Geometry: see drawing. Coordinates: mm, zero at the bounding-box minimum. Round coordinates to 2 decimals unless told otherwise and drop trailing zeros. Loops run counter-clockwise (first coordinate to the right, second up) from the corner with the lowest first, then second, coordinate; pieces in that order, holes last. Notation, with made-up numbers: (73, 59) - (107, 59) arc R24 ccw to (107, 70) - close; hole circle Ø9 at (18, -28.75). An arc over 180 degrees is marked (long way). Use CSV: the item, a comma, the result in double quotes. Start each with the question number.
1. Cut plane B-B (x = 3.25). Return loops of the section in (y, z) (1 decimal).
2. Pull-direction query (Y, two-part tool) for the marked faces 1, 2 and 3; classes: +Y half, -Y half, draft (parallel to the pull), parting line (faces both ways), or undercut.
3. Material intervals for probe 1 along Y at (x, z) = (2.5, 1.1); probe 2 along Y at (x, z) = (1.8, 1.95) (1 decimal); probe 3 along X at (y, z) = (32.5, 1.4), sorted ascending. Write a range as from..to.
4. Cut plane C-C (y = 31.5). Return loops of the section in (x, z).
5. Cut plane A-A (z = 0.95). Give the number of separate pieces and of enclosed holes in the cut face, and give its area (3 significant figures).
6. Cut plane D-D (y = 2). Return loops of the section in (x, z).
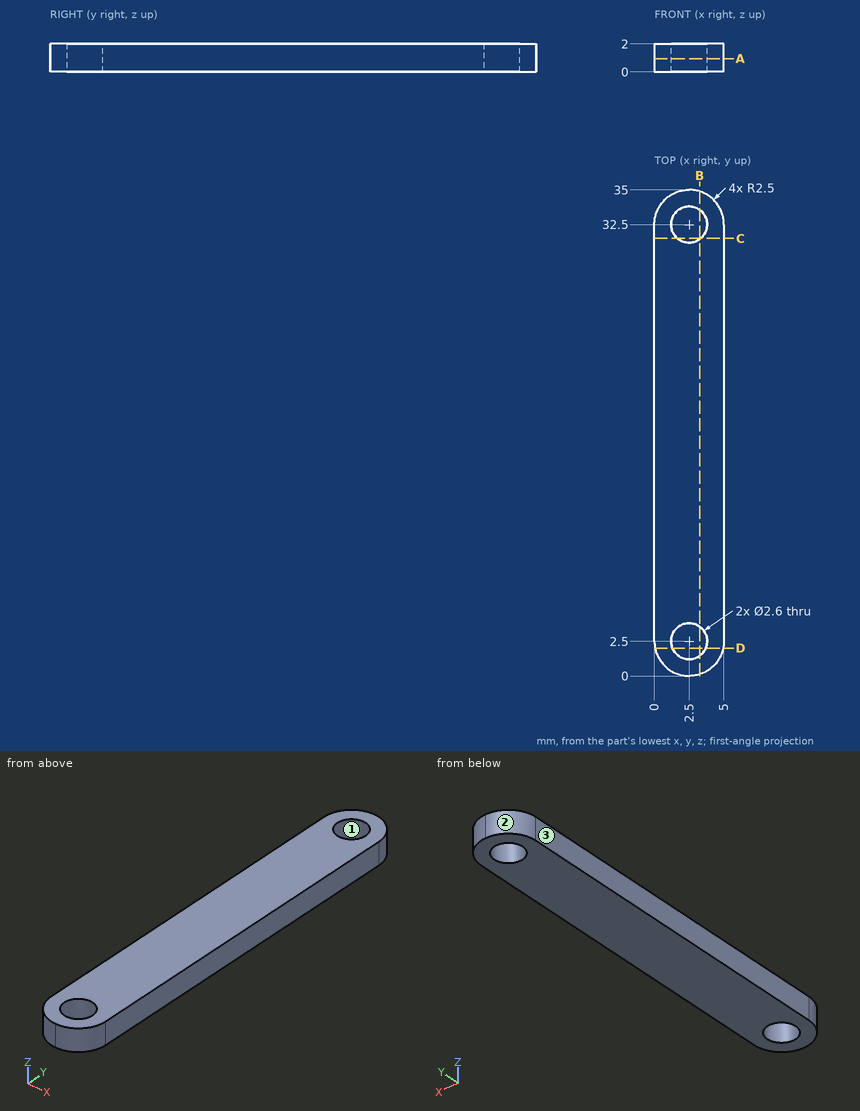
Established:
1,outline,"(0.1, 0) - (1.4, 0) - (1.4, 2) - (0.1, 2) - close; (3.6, 0) - (31.4, 0) - (31.4, 2) - (3.6, 2) - close; (33.6, 0) - (34.9, 0) - (34.9, 2) - (33.6, 2) - close"
2,face 1,"undercut"
2,face 2,"+Y half"
2,face 3,"draft"
3,probe 1,"y = 0..1.2, 3.8..31.2, 33.8..35"
3,probe 2,"y = 0.1..1.4, 3.6..31.4, 33.6..34.9"
3,probe 3,"x = 0..1.2, 3.8..5"
4,outline,"(0, 0) - (1.67, 0) - (1.67, 2) - (0, 2) - close; (3.33, 0) - (5, 0) - (5, 2) - (3.33, 2) - close"
5,separate pieces,"1"
5,enclosed holes,"2"
5,area,"159 mm2"
6,outline,"(0.05, 0) - (1.3, 0) - (1.3, 2) - (0.05, 2) - close; (3.7, 0) - (4.95, 0) - (4.95, 2) - (3.7, 2) - close"
